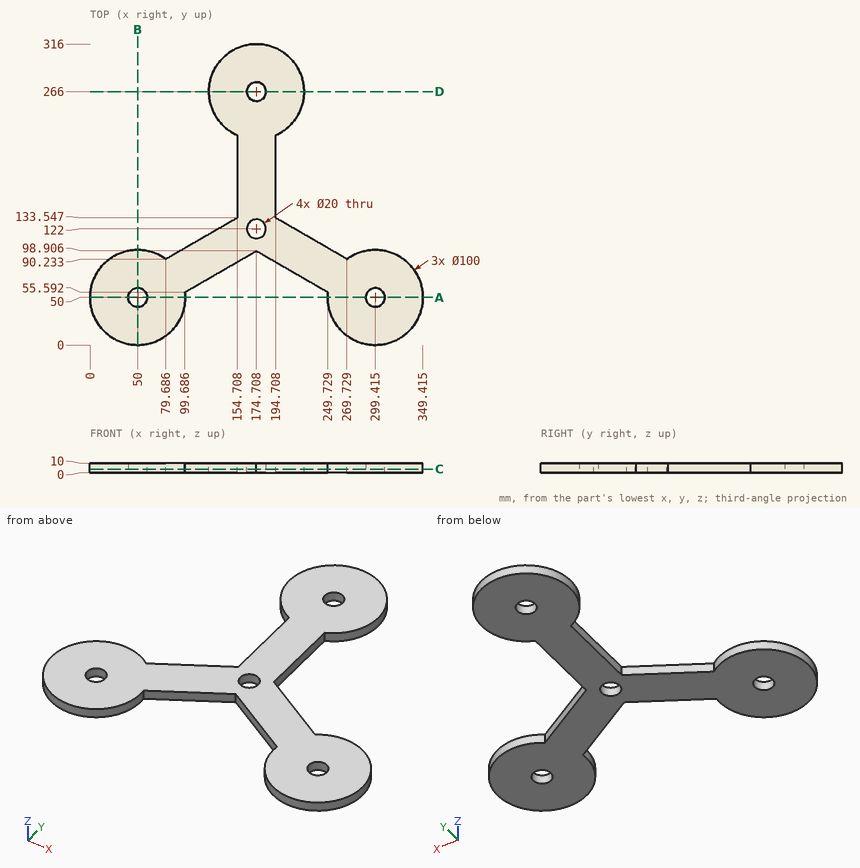
The drawing under review shows one solid part. Ordinate dimensions are in mm from its lowest x, y, z. Give positions to 0.01 mm unless a question says otherwise; leave off trailing zeros. Loops run counter-clockwise (first coordinate to the right, second up) from the corner with the lowest first, then second, coordinate; pieces in that order, holes last. Notation, with made-up numbers: M 48.25,-11.75 L 54.25,-11.75 A29 cw 54.25,16.25 Z; hole C 17.5,87 d5. An arc over 180 degrees is marked long. One line per item, written item: value. Start each with the question number.
Q1. Add section C-C (z = 3.75). Give the boundary of the cut face in (x, y) (1 decimal).
Q2. For L1, parallel to X at y = 50, z = 3 (1 decimal); L2, parallel to Y at x = 50, z = 3.5; L3, parallel to X at y = 266, z = 5, list the stretches that pass through material, from the lowest coordinate up.
Q3. Add section D-D (y = 266). Give the boundary of the cut face in (x, z).
Q4. Clearance check with flat-ended pins moving along their axes: pin 1 Ø4 at (x, z) = (218, 1.5) entering from +Y (1 decimal); pin 2 Ø5 at (y, z) = (53, 2) entering from -X; pin 3 Ø6 at (x, z) = (189, 2) entering from -Y; pin 4 Ø23 at (x, y) = (50, 50) entering from -Z. State where each tip first meets the part, or that it passes through.
Q5. Add section B-B (x = 50). Give the boundary of the cut face in (y, z).
Q6. Add section A-A (y = 50). Give the boundary of the cut face in (x, z) (1 decimal).
Reply:
1. outline: M 79.7,90.2 A50 ccw long 99.7,55.6 L 174.7,98.9 L 249.7,55.6 A50 ccw long 269.7,90.2 L 194.7,133.5 L 194.7,220.2 A50 ccw long 154.7,220.2 L 154.7,133.5 Z; hole C 50,50 d20; hole C 174.7,122 d20; hole C 174.7,266 d20; hole C 299.4,50 d20
2. L1: 0 to 40, 60 to 100, 249.4 to 289.4, 309.4 to 349.4
2. L2: 0 to 40, 60 to 100
2. L3: 124.71 to 164.71, 184.71 to 224.71
3. outline: M 124.71,0 L 164.71,0 L 164.71,10 L 124.71,10 Z; M 184.71,0 L 224.71,0 L 224.71,10 L 184.71,10 Z
4. pin 1: y = 294.2
4. pin 2: x = 0
4. pin 3: y = 88.92
4. pin 4: z = 0
5. outline: M 0,0 L 40,0 L 40,10 L 0,10 Z; M 60,0 L 100,0 L 100,10 L 60,10 Z
6. outline: M 0,0 L 40,0 L 40,10 L 0,10 Z; M 60,0 L 100,0 L 100,10 L 60,10 Z; M 249.4,0 L 289.4,0 L 289.4,10 L 249.4,10 Z; M 309.4,0 L 349.4,0 L 349.4,10 L 309.4,10 Z
